Geometry: final body of the model. Coordinates: model frame, mm. A direction names the side the tool comes from. Round coordinates to 2 decimals unless told otherwise and drop trailing zeros. Order: outer loops, then holes, each group sorted by start corner. A loop starts at its lowest first (then second) coordinate and runs counter-clockwise, first axis right, second up. Notation, with made-up numbers: (83, -24.5) - (126, -24.5) arc R22 cw to (126, 8.5) - close; hole circle Ø4 at (80, 42). An arc over 180 degrees is marked (long way). Put each result on its own line as item: value. Start each with the question number.
(1) Section D-D (z = 10). Output: boundary loops of the cut face in (x, y), and give its area (3 significant figures).
(2) Pin query (flat end, axial travel): P1, Ø1, axis at x = 33, y = 25.5, coming from the +Z side; P2, Ø6.5, axis at x = 13, y = 15, coming from the -Z side; P3, Ø7.5, axis at x = 19.05, z = 14.29, coming from the -Y side. Return the tip coordinate at first contact, or that it passes through.
(3) Section A-A (z = 37.5). Output: boundary loops of the cut face in (x, y), and give its area (3 significant figures).
(4) Section B-B (y = 6). Output: boundary loops of the cut face in (x, z), and give its area (3 significant figures).
(5) Material intervals for L1, parallel to Y at x = 30, z = 51; L2, parallel to Z at x = 19.05, y = 29.45; L3, parallel to Z at x = 14, y = 7, sorted ascending. Write a range as [from, to].
(6) Access query for faces 4 (the face through (38.1, -2, 50)), 5 (the face through (19, -1.588, 34)). Directions: +Z, -Z, +X, -X, +Y, -Y. A direction counts if a zero-diameter tool reaches every point of the face in a straight line with its end or side. Return the directions, or none.
(7) Pull-direction query (Y, two-part tool) for faces 1 (the face through (19.738, -3.153, 52.463)), 2 (the face through (19, 30.162, 34)), 3 (the face through (19.317, 26.033, 76.882)); classes: released by +Y, released by -Y, zero draft, split by the parting line, or undercut.
from build123d import *

# Parameters (mm, degrees)
F1_DEPTH = 38.1
F2_R     = 3.175
F3_R     = 6.35
F4_R     = 19.04999
F5_R     = 3.175
F6_DEPTH = 34.926


# Not quite as in the source:
# - a fillet or chamfer is up to 0.001 mm smaller than in the source, because OpenCascade refuses the exact size


with BuildPart() as f1:
    # F0 (on Right) → F1 (new body)
    with BuildSketch(Plane.YZ):
        Polygon((-1.5875, -4.7625), (-1.5875, 77.7875), (26.9875, 77.7875), (26.9875, -4.7625), (30.1625, -4.7625), (30.1625, 80.9625), (-4.7625, 80.9625), (-4.7625, -4.7625), align=None)
    extrude(amount=F1_DEPTH)

    # F2
    f2_edges = [f1.edges().sort_by_distance(p)[0] for p in [
        (19.05, 26.9875, 77.7875),
        (19.05, -1.5875, 77.7875),
    ]]
    fillet(f2_edges, radius=F2_R)

    # F3
    f3_edges = [f1.edges().sort_by_distance(p)[0] for p in [
        (19.05, 30.1625, 80.9625),
        (19.05, -4.7625, 80.9625),
    ]]
    fillet(f3_edges, radius=F3_R)

    # F4 (radius 19.05 in the source; OpenCascade refuses exactly that, so slightly less here)
    f4_edges = [f1.edges().sort_by_distance(p)[0] for p in [
        (38.1, 28.575, -4.7625),
        (0, 28.575, -4.7625),
        (38.1, -3.175, -4.7625),
        (0, -3.175, -4.7625),
    ]]
    fillet(f4_edges, radius=F4_R)

    # F5 (on face) → F6 (cut, through all)
    with BuildSketch(Plane(origin=(0, 30.1625, 0), x_dir=(-1, 0, 0), z_dir=(0, 1, 0))):
        with Locations((-19.05, 14.2875)):
            Circle(F5_R)
        with Locations((-19.05, 55.5625)):
            Circle(F5_R)
    extrude(amount=-F6_DEPTH, mode=Mode.SUBTRACT)


solid = f1.part
Checks:
1. outline: (0.49, -4.76) - (37.61, -4.76) - (37.61, -1.59) - (0.49, -1.59) - close; (0.49, 26.99) - (37.61, 26.99) - (37.61, 30.16) - (0.49, 30.16) - close
1. area: 236 mm²
2. P1: stops at z = 80.85
2. P2: stops at z = 77.79
2. P3: stops at y = -4.76
3. outline: (0, -4.76) - (38.1, -4.76) - (38.1, -1.59) - (0, -1.59) - close; (0, 26.99) - (38.1, 26.99) - (38.1, 30.16) - (0, 30.16) - close
3. area: 242 mm²
4. outline: (0, 77.79) - (38.1, 77.79) - (38.1, 80.96) - (0, 80.96) - close
4. area: 121 mm²
5. L1: y = [-4.76, -1.59], [26.99, 30.16]
5. L2: z = [-4.76, 11.11], [17.46, 52.39], [58.74, 77.54]
5. L3: z = [77.79, 80.96]
6. face 4: +Z, -Z, +X, +Y, -Y
6. face 5: -Z, +X, -X
7. face 1: zero draft
7. face 2: released by +Y
7. face 3: undercut
